Design review of the part built by this model. Coordinates are the model's own, in mm. A direction names the side the tool comes from. Give positions to 0.01 mm unless a question says otherwise; leave off trailing zeros. Write each loop counter-clockwise with the first axis right and the second up, starting at its lowest first coordinate (ties: lowest second). Pieces come first, ordered by that corner, then holes. Notation, with made-up numbers: (65.25, -14.5) - (111.25, -14.5) arc R20 cw to (111.25, -9.5) - close; hole circle Ø7 at (63.5, 11.25). An arc over 180 degrees is marked (long way). Use a Markdown table: item, result. Add a question column.
```python
from build123d import *

# Parameters (mm, degrees)
SKETCH1_R           = 80
SKETCH1_R_2         = 6
BOSS_EXTRUDE1_DEPTH = 18
SKETCH2_R           = 65
SKETCH2_R_2         = 13
CUT_EXTRUDE1_DEPTH  = 13
CUT_EXTRUDE3_DEPTH  = 24
CHAMFER1_SIZE       = 1
SKETCH4_R           = 2.5
CUT_EXTRUDE4_DEPTH  = 13


with BuildPart() as part:
    # Sketch1 → Boss-Extrude1 (new body, symmetric)
    with BuildSketch(Plane.XY):
        Circle(SKETCH1_R)
        Circle(SKETCH1_R_2, mode=Mode.SUBTRACT)
    extrude(amount=BOSS_EXTRUDE1_DEPTH, both=True)

    # Sketch2 → Cut-Extrude1 (cut)
    with BuildSketch(Plane.XY.offset(18)):
        Circle(SKETCH2_R)
        Circle(SKETCH2_R_2, mode=Mode.SUBTRACT)
    cut_extrude1 = extrude(amount=-CUT_EXTRUDE1_DEPTH, mode=Mode.SUBTRACT)

    # Mirror1: Cut-Extrude1 across plane
    add(cut_extrude1.mirror(Plane.XY), mode=Mode.SUBTRACT)

    # Sketch3 → Cut-Extrude3 (cut, through all)
    with BuildSketch(Plane.XY.offset(5)):
        with BuildLine():
            Line((0, 19.397164741), (0, 54.772255751))
            ThreePointArc((0, 54.772255751), (-1.629000688, 58.46500048), (-5.454545455, 59.751551728))
            ThreePointArc((-5.454545455, 59.751551728), (-15.529142706, 57.955549577), (-25.152000934, 54.473634439))
            ThreePointArc((-25.152000934, 54.473634439), (-27.821744262, 51.446675992), (-27.386127875, 47.434164903))
            Line((-27.386127875, 47.434164903), (-9.698582371, 16.798437427))
            ThreePointArc((-9.698582371, 16.798437427), (-8.582686936, 15.895715021), (-7.149451403, 15.972956666))
            ThreePointArc((-7.149451403, 15.972956666), (-4.529333289, 16.90370196), (-1.794871795, 17.407711947))
            ThreePointArc((-1.794871795, 17.407711947), (-0.515032591, 18.057436487), (0, 19.397164741))
        make_face()
        with BuildLine():
            Line((2.027555822, 19.290905043), (5.725259723, 54.472207603))
            ThreePointArc((5.725259723, 54.472207603), (7.731333507, 57.974446151), (11.670402764, 58.854071221))
            ThreePointArc((11.670402764, 58.854071221), (21.502076973, 56.01482559), (30.708260938, 51.546122164))
            ThreePointArc((30.708260938, 51.546122164), (33.046975817, 48.256681545), (32.194324165, 44.311685722))
            Line((32.194324165, 44.311685722), (11.401367371, 15.692635918))
            ThreePointArc((11.401367371, 15.692635918), (10.197224742, 14.911501555), (8.779914574, 15.138133969))
            ThreePointArc((8.779914574, 15.138133969), (6.271439117, 16.337657464), (3.604640678, 17.124735489))
            ThreePointArc((3.604640678, 17.124735489), (2.399727275, 17.904680395), (2.027555822, 19.290905043))
        make_face()
        with BuildLine():
            Line((12.979236605, 14.414902606), (36.649792702, 40.703718441))
            ThreePointArc((36.649792702, 40.703718441), (40.331304654, 42.35794836), (44.035109268, 40.754253173))
            ThreePointArc((44.035109268, 40.754253173), (50.320234077, 32.678342101), (55.141555387, 23.651825922))
            ThreePointArc((55.141555387, 23.651825922), (55.100130785, 19.615950443), (52.091510744, 16.925557847))
            Line((52.091510744, 16.925557847), (18.447799925, 5.994053548))
            ThreePointArc((18.447799925, 5.994053548), (17.014488815, 6.069879851), (16.001071994, 7.086303341))
            ThreePointArc((16.001071994, 7.086303341), (14.676734939, 9.531183113), (12.981882537, 11.735447405))
            ThreePointArc((12.981882537, 11.735447405), (12.465527231, 13.074666417), (12.979236605, 14.414902606))
        make_face()
        with BuildLine():
            Line((18.973290153, 4.032897318), (53.575350549, 11.387792303))
            ThreePointArc((53.575350549, 11.387792303), (57.526088234, 10.562153989), (59.579900731, 7.087695599))
            ThreePointArc((59.579900731, 7.087695599), (59.917772085, -3.140157375), (58.512649872, -13.276663926))
            ThreePointArc((58.512649872, -13.276663926), (56.106908578, -16.517407005), (52.091510744, -16.925557847))
            Line((52.091510744, -16.925557847), (18.447799925, -5.994053548))
            ThreePointArc((18.447799925, -5.994053548), (17.332796462, -5.090229647), (17.110363769, -3.672254308))
            ThreePointArc((17.110363769, -3.672254308), (17.476016858, -0.915879234), (17.400486505, 1.863617284))
            ThreePointArc((17.400486505, 1.863617284), (17.769919472, 3.250574258), (18.973290153, 4.032897318))
        make_face()
        with BuildLine():
            Line((17.720191741, -7.889537672), (50.036945446, -22.277883438))
            ThreePointArc((50.036945446, -22.277883438), (52.747861348, -25.268024211), (52.36719516, -29.286120792))
            ThreePointArc((52.36719516, -29.286120792), (46.628757687, -37.759223463), (39.533900877, -45.133919412))
            ThreePointArc((39.533900877, -45.133919412), (35.682754298, -46.341676384), (32.194324165, -44.311685722))
            Line((32.194324165, -44.311685722), (11.401367371, -15.692635918))
            ThreePointArc((11.401367371, -15.692635918), (11.03056498, -14.306044431), (11.684078144, -13.028135628))
            ThreePointArc((11.684078144, -13.028135628), (13.600054325, -11.013106843), (15.172696049, -8.720051296))
            ThreePointArc((15.172696049, -8.720051296), (16.286806452, -7.815126784), (17.720191741, -7.889537672))
        make_face()
        with BuildLine():
            Line((9.698582371, -16.798437427), (27.386127875, -47.434164903))
            ThreePointArc((27.386127875, -47.434164903), (27.821744262, -51.446675992), (25.152000934, -54.473634439))
            ThreePointArc((25.152000934, -54.473634439), (15.529142706, -57.955549577), (5.454545455, -59.751551728))
            ThreePointArc((5.454545455, -59.751551728), (1.629000688, -58.46500048), (0, -54.772255751))
            Line((0, -54.772255751), (0, -19.397164741))
            ThreePointArc((0, -19.397164741), (0.515032591, -18.057436487), (1.794871795, -17.407711947))
            ThreePointArc((1.794871795, -17.407711947), (4.529333289, -16.90370196), (7.149451403, -15.972956666))
            ThreePointArc((7.149451403, -15.972956666), (8.582686936, -15.895715021), (9.698582371, -16.798437427))
        make_face()
        with BuildLine():
            Line((-2.027555822, -19.290905043), (-5.725259723, -54.472207603))
            ThreePointArc((-5.725259723, -54.472207603), (-7.731333507, -57.974446151), (-11.670402764, -58.854071221))
            ThreePointArc((-11.670402764, -58.854071221), (-21.502076973, -56.01482559), (-30.708260938, -51.546122164))
            ThreePointArc((-30.708260938, -51.546122164), (-33.046975817, -48.256681545), (-32.194324165, -44.311685722))
            Line((-32.194324165, -44.311685722), (-11.401367371, -15.692635918))
            ThreePointArc((-11.401367371, -15.692635918), (-10.197224742, -14.911501555), (-8.779914574, -15.138133969))
            ThreePointArc((-8.779914574, -15.138133969), (-6.271439117, -16.337657464), (-3.604640678, -17.124735489))
            ThreePointArc((-3.604640678, -17.124735489), (-2.399727275, -17.904680395), (-2.027555822, -19.290905043))
        make_face()
        with BuildLine():
            Line((-12.979236605, -14.414902606), (-36.649792702, -40.703718441))
            ThreePointArc((-36.649792702, -40.703718441), (-40.331304654, -42.35794836), (-44.035109268, -40.754253173))
            ThreePointArc((-44.035109268, -40.754253173), (-50.320234077, -32.678342101), (-55.141555387, -23.651825922))
            ThreePointArc((-55.141555387, -23.651825922), (-55.100130785, -19.615950443), (-52.091510744, -16.925557847))
            Line((-52.091510744, -16.925557847), (-18.447799925, -5.994053548))
            ThreePointArc((-18.447799925, -5.994053548), (-17.014488815, -6.069879851), (-16.001071994, -7.086303341))
            ThreePointArc((-16.001071994, -7.086303341), (-14.676734939, -9.531183113), (-12.981882537, -11.735447405))
            ThreePointArc((-12.981882537, -11.735447405), (-12.465527231, -13.074666417), (-12.979236605, -14.414902606))
        make_face()
        with BuildLine():
            Line((-18.973290153, -4.032897318), (-53.575350549, -11.387792303))
            ThreePointArc((-53.575350549, -11.387792303), (-57.526088234, -10.562153989), (-59.579900731, -7.087695599))
            ThreePointArc((-59.579900731, -7.087695599), (-59.917772085, 3.140157375), (-58.512649872, 13.276663926))
            ThreePointArc((-58.512649872, 13.276663926), (-56.106908578, 16.517407005), (-52.091510744, 16.925557847))
            Line((-52.091510744, 16.925557847), (-18.447799925, 5.994053548))
            ThreePointArc((-18.447799925, 5.994053548), (-17.332796462, 5.090229647), (-17.110363769, 3.672254308))
            ThreePointArc((-17.110363769, 3.672254308), (-17.476016858, 0.915879234), (-17.400486505, -1.863617284))
            ThreePointArc((-17.400486505, -1.863617284), (-17.769919472, -3.250574258), (-18.973290153, -4.032897318))
        make_face()
        with BuildLine():
            Line((-17.720191741, 7.889537672), (-50.036945446, 22.277883438))
            ThreePointArc((-50.036945446, 22.277883438), (-52.747861348, 25.268024211), (-52.36719516, 29.286120792))
            ThreePointArc((-52.36719516, 29.286120792), (-46.628757687, 37.759223463), (-39.533900877, 45.133919412))
            ThreePointArc((-39.533900877, 45.133919412), (-35.682754298, 46.341676384), (-32.194324165, 44.311685722))
            Line((-32.194324165, 44.311685722), (-11.401367371, 15.692635918))
            ThreePointArc((-11.401367371, 15.692635918), (-11.03056498, 14.306044431), (-11.684078144, 13.028135628))
            ThreePointArc((-11.684078144, 13.028135628), (-13.600054325, 11.013106843), (-15.172696049, 8.720051296))
            ThreePointArc((-15.172696049, 8.720051296), (-16.286806452, 7.815126784), (-17.720191741, 7.889537672))
        make_face()
    extrude(amount=-CUT_EXTRUDE3_DEPTH, mode=Mode.SUBTRACT)

    # Chamfer1
    chamfer1_edges = [part.edges().sort_by_distance(p)[0] for p in [
        (-65, 0, -18),
        (-80, 0, 18),
    ]]
    chamfer(chamfer1_edges, length=CHAMFER1_SIZE)

    # Sketch4 → Cut-Extrude4 (cut, symmetric)
    with BuildSketch(Plane(origin=(0, 0, 0), x_dir=(1, 0, 0), z_dir=(0, 1, 0))):
        with Locations((0, -12)):
            Circle(SKETCH4_R)
    extrude(amount=CUT_EXTRUDE4_DEPTH, both=True, mode=Mode.SUBTRACT)


solid = part.part
```
(1) Tool access review of faces 1 (the face through (2.31, 9.28, 12.96)), 2 (the face through (-40.273, -42.357, 0.07)), 3 (the face through (62, 19.52, 11.59)): name each direction out of +Z, -Z, +X, -X, +Y, -Y from which nothing blocks a thin tool from reaching the whole face with its end or side.
(2) Insertion check: pin 1 (5 mm diameter, centred on y = -32, z = -2, fed in from +X); pin 2 (1.5 mm diameter, centred on y = -63, z = 14.5, fed in from +X); pin 3 (4 mm diameter, centred on x = -48, z = 0, fed in from +Y); pin 4 (2 mm diameter, centred on x = 30, y = 45.5, fed in from +Z). Each pin has a flat end and moves straight along its axis. Give the tip position at first contact, or say it passes through.
(3) Add section A-A (z = 12). State the section outline as (x, y) points.
(4) Add section B-B (y = 0). Count the separate pieces of the cut face and the enclosed holes in it, and give its area (3 significant figures).
(5) For line 1 along Y through (x, z) = (0, -8.5); line 2 along Z through (x, y) = (0, 11.75); line 3 along Y through (x, z) = (-3, -7), list the stretches that pass through material, from the lowest coordinate up.
Answers follow:
| question | item | result |
|---|---|---|
| 1 | face 1 | none |
| 1 | face 2 | +Z, -Z |
| 1 | face 3 | +Z |
| 2 | pin 1 | x = 74.36 |
| 2 | pin 2 | x = 50.25 |
| 2 | pin 3 | y = 65.45 |
| 2 | pin 4 | through |
| 3 | outline | circle Ø160 at (0, 0); (-2.5, -12.76) - (-2.5, -5.45) arc R6 cw to (-2.5, 5.45) - (-2.5, 12.76) arc R13 ccw to start; (2.5, -12.76) arc R13 ccw to (2.5, 12.76) - (2.5, 5.45) arc R6 cw to (2.5, -5.45) - close; hole circle Ø130 at (0, 0) |
| 4 | separate pieces | 4 |
| 4 | enclosed holes | 0 |
| 4 | area | 1,770 mm^2 |
| 5 | line 1 | -80 to -65, -13 to -6, 6 to 13, 65 to 80 |
| 5 | line 2 | -18 to 9.5, 14.5 to 18 |
| 5 | line 3 | -79.94 to -64.93, -12.65 to -5.2, 5.2 to 12.65, 64.93 to 79.94 |
